from build123d import *

# Parameters (mm, degrees)
SKETCH_1_W          = 20
SKETCH_1_H          = 60
EXTRUDE_1_DEPTH     = 4.5
SKETCH_2_W          = 20
SKETCH_2_H          = 20
EXTRUDE_2_DEPTH     = 40
SKETCH_3_W          = 100
SKETCH_3_H          = 20
EXTRUDE_3_DEPTH     = 5
SKETCH_5_R          = 2.5
CUT_EXTRUDE_2_DEPTH = 5
SKETCH_6_R          = 2.55
CUT_EXTRUDE_3_DEPTH = 10


with BuildPart() as part:
    # 草图1 → 凸台-拉伸1 (new body)
    with BuildSketch(Plane.XY):
        Rectangle(SKETCH_1_W, SKETCH_1_H)
    extrude(amount=EXTRUDE_1_DEPTH)

    # 草图2 → 凸台-拉伸2 (add)
    with BuildSketch(Plane.XY.offset(4.5)):
        Rectangle(SKETCH_2_W, SKETCH_2_H)
    extrude(amount=EXTRUDE_2_DEPTH)

    # 草图3 → 凸台-拉伸3 (add)
    with BuildSketch(Plane.XY.offset(44.5)):
        with Locations((40, 0)):
            Rectangle(SKETCH_3_W, SKETCH_3_H)
    extrude(amount=EXTRUDE_3_DEPTH)

    # 草图5 → 切除-拉伸2 (cut)
    with BuildSketch(Plane.XY.offset(4.5)):
        with Locations((0, 20)):
            Circle(SKETCH_5_R)
        with Locations((0, -20)):
            Circle(SKETCH_5_R)
    extrude(amount=-CUT_EXTRUDE_2_DEPTH, mode=Mode.SUBTRACT)

    # 草图6 → 切除-拉伸3 (cut)
    with BuildSketch(Plane.XY.offset(49.5)):
        with Locations((80, 0)):
            Circle(SKETCH_6_R)
        with Locations((68, 0)):
            Circle(SKETCH_6_R)
        with Locations((56, 0)):
            Circle(SKETCH_6_R)
    extrude(amount=-CUT_EXTRUDE_3_DEPTH, mode=Mode.SUBTRACT)


solid = part.part
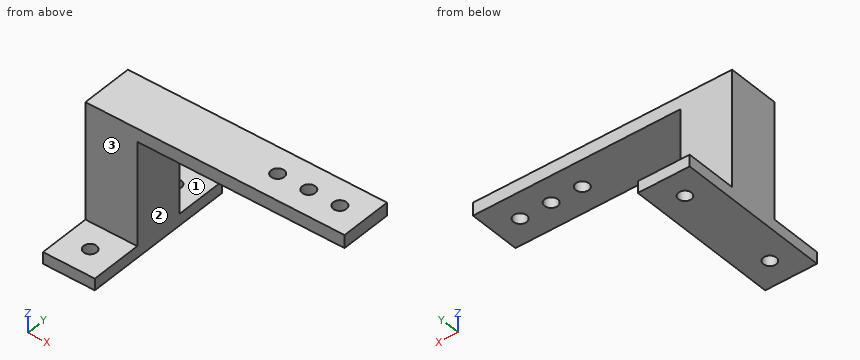
Build history of the part. All positions in model axes, mm. Face numbers are marked on the shaded views. A direction names the side the tool comes from. Round coordinates to 2 decimals unless told otherwise and drop trailing zeros. Write each loop counter-clockwise with the first axis right and the second up, starting at its lowest first coordinate (ties: lowest second). Pieces come first, ordered by that corner, then holes. Notation, with made-up numbers: (27, 24) -> (86, 24) arc R21 cw to (86, 45) -> close; hole circle Ø6 at (24, 34.25). An arc over 180 degrees is marked (long way). Use one line per item in the form item = value.
Q1. Drop flat-ended pins along their axis: P1, Ø4.5, axis at x = 0, y = -20, coming from the +Z side; P2, Ø16, axis at x = 3, y = -23, coming from the +Z side; P3, Ø8, axis at x = 56, y = 0, coming from the -Z side; P4, Ø12, axis at x = 60, z = 39.5, coming from the -Y side. Give the stop position or say it passes through.
Conclusion:
P1 = through
P2 = 4.5
P3 = 44.5
P4 = -10
Q2. Band-saw the part on C-C, the plane x = 68. Write the cut outline in (y, z).
Conclusion:
outline = (-10, 44.5) -> (-2.55, 44.5) -> (-2.55, 49.5) -> (-10, 49.5) -> close; (2.55, 44.5) -> (10, 44.5) -> (10, 49.5) -> (2.55, 49.5) -> close
Q3. Band-saw the part on D-D, the plane y = 0. Write the cut outline in (x, z).
Conclusion:
outline = (-10, 0) -> (10, 0) -> (10, 44.5) -> (53.45, 44.5) -> (53.45, 49.5) -> (-10, 49.5) -> close; (58.55, 44.5) -> (65.45, 44.5) -> (65.45, 49.5) -> (58.55, 49.5) -> close; (70.55, 44.5) -> (77.45, 44.5) -> (77.45, 49.5) -> (70.55, 49.5) -> close; (82.55, 44.5) -> (90, 44.5) -> (90, 49.5) -> (82.55, 49.5) -> close
Q4. Band-saw the part on A-A, the plane x = 0. Write the cut outline in (y, z), then the cut area to 4 significant figures.
Conclusion:
outline = (-30, 0) -> (-22.5, 0) -> (-22.5, 4.5) -> (-30, 4.5) -> close; (-17.5, 0) -> (17.5, 0) -> (17.5, 4.5) -> (10, 4.5) -> (10, 49.5) -> (-10, 49.5) -> (-10, 4.5) -> (-17.5, 4.5) -> close; (22.5, 0) -> (30, 0) -> (30, 4.5) -> (22.5, 4.5) -> close
area = 1,125 mm²
Q5. Drill centre lines: L1, parallel to Y at x = 0, z = 2.55; L2, parallel to Y at x = 68, z = 45; L3, parallel to X at y = -1, z = 16. Where is each one in solid material? Low to high.
Conclusion:
L1 = -30 to -22.5, -17.5 to 17.5, 22.5 to 30
L2 = -10 to -2.55, 2.55 to 10
L3 = -10 to 10
Q6. Band-saw the part on B-B, the plane y = -20. Write the cut outline in (x, z), then the cut area to 3 significant figures.
Conclusion:
outline = (-10, 0) -> (-2.5, 0) -> (-2.5, 4.5) -> (-10, 4.5) -> close; (2.5, 0) -> (10, 0) -> (10, 4.5) -> (2.5, 4.5) -> close
area = 67.5 mm²
Q7. Tool access for the marked faces 1, 2 and 3: list every direction of +Z, -Z, +X, -X, +Y, -Y with a clear straight run to the whole face (end or side of a thin tool).
Conclusion:
face_1 = +Z, +X, -X, +Y
face_2 = -Z, +X, +Y, -Y
face_3 = +Z, +X, -X, -Y
